Can you work these out from the model? Positions are in its coordinate system, mm. Round coordinates to 2 decimals unless told otherwise and drop trailing zeros. Order: outer loops, then holes, each group sorted by start corner. A loop starts at its lowest first (then second) coordinate and runs counter-clockwise, first axis right, second up. Notation, with made-up numbers: (56.5, -39) -> (74.5, -39) arc R23 cw to (74.5, -14) -> close; hole circle Ø1 at (71.5, 52.25). An arc over 180 degrees is marked (long way). One line per item, written item: value.
```python
from build123d import *

# Parameters (mm, degrees)
BOSS_EXTRUDE1_DEPTH  = 18
SKETCH4_R            = 3
CUT_EXTRUDE2_DEPTH   = 30
M3_CLEARANCE_HOLE1_D = 3.4


with BuildPart() as part:
    # Sketch1 → Boss-Extrude1 (new body)
    with BuildSketch(Plane.XY):
        Polygon((-961.236516538, 328.950735931), (-961.236516538, 378.950735931), (-943.236516538, 378.950735931), (-943.236516538, 657.901471863), (-961.236516538, 657.901471863), (-961.236516538, 707.901471863), (-943.236516538, 707.901471863), (-943.236516538, 807.901471863), (-843.236516538, 807.901471863), (-843.236516538, 825.901471863), (-793.236516538, 825.901471863), (-793.236516538, 807.901471863), (-439.118258269, 807.901471863), (-439.118258269, 825.901471863), (-389.118258269, 825.901471863), (-389.118258269, 807.901471863), (-35, 807.901471863), (-35, 825.901471863), (15, 825.901471863), (15, 807.901471863), (115, 807.901471863), (115, 707.901471863), (133, 707.901471863), (133, 657.901471863), (115, 657.901471863), (115, 378.950735931), (133, 378.950735931), (133, 328.950735931), (115, 328.950735931), (115, 50), (133, 50), (133, 0), (115, 0), (115, -100), (15, -100), (15, -118), (-35, -118), (-35, -100), (-389.118258269, -100), (-389.118258269, -118), (-439.118258269, -118), (-439.118258269, -100), (-793.236516538, -100), (-793.236516538, -118), (-843.236516538, -118), (-843.236516538, -100), (-943.236516538, -100), (-943.236516538, 0), (-961.236516538, 0), (-961.236516538, 50), (-943.236516538, 50), (-943.236516538, 328.950735931), align=None)
    extrude(amount=BOSS_EXTRUDE1_DEPTH)

    # Sketch4 → Cut-Extrude2 (cut)
    with BuildSketch(Plane.XY.offset(18)):
        with Locations((-845.357836881, 810.022792206)):
            Circle(SKETCH4_R)
        with Locations((-791.115196194, 810.022792206)):
            Circle(SKETCH4_R)
        with Locations((-37.121320344, 810.022792206)):
            Circle(SKETCH4_R)
        with Locations((17.121320344, 810.022792206)):
            Circle(SKETCH4_R)
        with Locations((-441.239578612, 810.022792206)):
            Circle(SKETCH4_R)
        with Locations((-386.996937925, 810.022792206)):
            Circle(SKETCH4_R)
        with Locations((-386.996937925, -102.121320344)):
            Circle(SKETCH4_R)
        with Locations((-441.239578612, -102.121320344)):
            Circle(SKETCH4_R)
        with Locations((17.121320344, -102.121320344)):
            Circle(SKETCH4_R)
        with Locations((-37.121320344, -102.121320344)):
            Circle(SKETCH4_R)
        with Locations((-791.115196194, -102.121320344)):
            Circle(SKETCH4_R)
        with Locations((-845.357836881, -102.121320344)):
            Circle(SKETCH4_R)
        with Locations((117.121320344, 381.072056275)):
            Circle(SKETCH4_R)
        with Locations((117.121320344, 326.829415588)):
            Circle(SKETCH4_R)
        with Locations((117.121320344, 710.022792206)):
            Circle(SKETCH4_R)
        with Locations((117.121320344, 655.780151519)):
            Circle(SKETCH4_R)
        with Locations((117.121320344, 52.121320344)):
            Circle(SKETCH4_R)
        with Locations((117.121320344, -2.121320344)):
            Circle(SKETCH4_R)
        with Locations((-945.357836881, -2.121320344)):
            Circle(SKETCH4_R)
        with Locations((-945.357836881, 52.121320344)):
            Circle(SKETCH4_R)
        with Locations((-945.357836881, 655.780151519)):
            Circle(SKETCH4_R)
        with Locations((-945.357836881, 710.022792206)):
            Circle(SKETCH4_R)
        with Locations((-945.357836881, 326.829415588)):
            Circle(SKETCH4_R)
        with Locations((-945.357836881, 381.072056275)):
            Circle(SKETCH4_R)
    extrude(amount=-CUT_EXTRUDE2_DEPTH, mode=Mode.SUBTRACT)

    # M3 Clearance Hole1 (through all)
    with Locations(Plane(origin=(0, 0, 0), x_dir=(-1, 0, 0), z_dir=(0, 0, -1))):
        with Locations((-124, 682.901471863), (-124, 353.950735931), (-124, 25), (10, -109), (414.118258269, -109), (818.236516538, -109), (952.236516538, 25), (952.236516538, 353.950735931), (952.236516538, 682.901471863), (818.236516538, 816.901471863), (414.118258269, 816.901471863), (10, 816.901471863)):
            Hole(M3_CLEARANCE_HOLE1_D / 2)


solid = part.part
```
Q1. I want a section at C-C on z = 10. Give the number of separate pieces and of enclosed holes in the cut face, plus the area to 3 significant figures.
Answers below:
separate pieces: 1
enclosed holes: 12
area: 971,000 mm^2
Q2. Please list where these lines run through material, in increasing order: line 1 along Y through (x, z) = (124, 9.5); line 2 along X through (y, z) = (-109, 9.5); line 3 along Y through (x, z) = (-875, 15.5).
Answers below:
line 1: 0 to 23.3, 26.7 to 50, 328.95 to 352.25, 355.65 to 378.95, 657.9 to 681.2, 684.6 to 707.9
line 2: -843.24 to -819.94, -816.54 to -793.24, -439.12 to -415.82, -412.42 to -389.12, -35 to -11.7, -8.3 to 15
line 3: -100 to 807.9
Q3. I want a section at B-B on x = -873.5. List the corners of the cut face in (y, z) for me.
Answers below:
outline: (-100, 0) -> (807.9, 0) -> (807.9, 18) -> (-100, 18) -> close
Q4. I want a section at A-A on y = 256. List the corners of the cut face in (x, z) for me, plus the area to 3 significant figures.
Answers below:
outline: (-943.24, 0) -> (115, 0) -> (115, 18) -> (-943.24, 18) -> close
area: 19,000 mm^2
Q5. Will these pins go through, and if not, where does the flat tip stop? pin 1 Ø4 at (y, z) = (819, 5) entering from -X; pin 2 Ø5.5 at (x, y) = (-818.24, 816.9) entering from -Z; pin 3 Ø9 at (y, z) = (754, 12) entering from +X; pin 4 Ø4 at (x, z) = (-957.5, 10) entering from -Y.
Answers below:
pin 1: x = -843.24
pin 2: z = 0
pin 3: x = 115
pin 4: y = 0
